```python
from build123d import *

# Parameters (mm, degrees)
SKETCH_1_W          = 22.5
SKETCH_1_H          = 17
EXTRUDE_1_DEPTH     = 6.5
SKETCH_2_W          = 7
SKETCH_2_H          = 3.2
CUT_EXTRUDE_1_DEPTH = 29.939592257
SKETCH_3_R          = 1
CUT_EXTRUDE_2_DEPTH = 2.4


with BuildPart() as part:
    # 草图1 → 凸台-拉伸1 (new body)
    with BuildSketch(Plane(origin=(0, 0, 0), x_dir=(1, 0, 0), z_dir=(0, 1, 0))):
        with Locations((11.25, 8.5)):
            Rectangle(SKETCH_1_W, SKETCH_1_H)
    extrude(amount=EXTRUDE_1_DEPTH)

    # 草图2 → 切除-拉伸1 (cut, through all)
    with BuildSketch(Plane.ZY):
        with Locations((-8.5, 1.6)):
            Rectangle(SKETCH_2_W, SKETCH_2_H)
    extrude(amount=-CUT_EXTRUDE_1_DEPTH, mode=Mode.SUBTRACT)

    # 草图3 → 切除-拉伸2 (cut)
    with BuildSketch(Plane(origin=(0, 6.5, 0), x_dir=(1, 0, 0), z_dir=(0, 1, 0))):
        with Locations(Location((7.25, 14.5, 0), (0, 0, 270))):
            Circle(SKETCH_3_R)
        with Locations(Location((15.25, 14.5, 0), (0, 0, 270))):
            Circle(SKETCH_3_R)
        with Locations(Location((15.25, 2.5, 0), (0, 0, 90))):
            Circle(SKETCH_3_R)
        with Locations(Location((7.25, 2.5, 0), (0, 0, 90))):
            Circle(SKETCH_3_R)
    extrude(amount=-CUT_EXTRUDE_2_DEPTH, mode=Mode.SUBTRACT)


solid = part.part
```
Geometry: final body of the model. Coordinates: model frame, mm. A direction names the side the tool comes from. Round coordinates to 2 decimals unless told otherwise and drop trailing zeros. Write each loop counter-clockwise with the first axis right and the second up, starting at its lowest first coordinate (ties: lowest second). Pieces come first, ordered by that corner, then holes. Notation, with made-up numbers: (74, 59) -> (94, 59) arc R28 cw to (94, 81) -> close; hole circle Ø3 at (80, 88). An arc over 180 degrees is marked (long way). Use CSV: the item, a comma, the result in double quotes. Start each with the question number.
Q1. Section D-D (x = 15.25). Return loops of the section in (y, z), plus the area to 3 significant figures.
Q2. First-contact query: pin 1 Ø2 at (x, z) = (14.5, -9) entering from -Y. Flat tip, straight axial feed; report the tip coordinate or a pass-through.
Q3. Section C-C (y = 0.75). Return loops of the section in (x, z), plus the area to 3 significant figures.
Q4. Reachability of faces 4 (the face through (15, 4.1, -2)), 5 (the face through (11, 2, -12)), 6 (the face through (11, 3, 0)) from +Z, -Z, +X, -X, +Y, -Y: full face, straight path, thin tool, end or side. Return the list, or none.
Q5. Line query: L1, parallel to X at y = 5, z = -14.5; L2, parallel to Z at x = 18.75, y = 0.75; L3, parallel to Y at x = 14.5, z = -3. Output: solid intervals per line, ascending.
Q6. Section B-B (z = -14.5). Return loops of the section in (x, y), plus the area to 3 significant figures.
Q7. Section A-A (y = 5.5). Return loops of the section in (x, z), plus the area to 3 significant figures.
Q8. Pull-direction query (X, two-part tool) for faces 1 (the face through (11, 3.2, -9)), 2 (the face through (7, 4.1, -15)), 3 (the face through (0, 4, -8)); classes: pulls with the +X half, pulls with the -X half, needs draft (parallel to the pull), parting line crosses it, or undercut.
Result sheet:
1,outline,"(0, -17) -> (6.5, -17) -> (6.5, -15.5) -> (4.1, -15.5) -> (4.1, -13.5) -> (6.5, -13.5) -> (6.5, -3.5) -> (4.1, -3.5) -> (4.1, -1.5) -> (6.5, -1.5) -> (6.5, 0) -> (0, 0) -> (0, -5) -> (3.2, -5) -> (3.2, -12) -> (0, -12) -> close"
1,area,"78.5 mm²"
2,pin 1,"y = 3.2"
3,outline,"(0, -17) -> (22.5, -17) -> (22.5, -12) -> (0, -12) -> close; (0, -5) -> (22.5, -5) -> (22.5, 0) -> (0, 0) -> close"
3,area,"225 mm²"
4,face 4,"+Y"
4,face 5,"+X, -X, -Y"
4,face 6,"+Z, +X, -X, +Y, -Y"
5,L1,"0 to 6.25, 8.25 to 14.25, 16.25 to 22.5"
5,L2,"-17 to -12, -5 to 0"
5,L3,"0 to 4.1"
6,outline,"(0, 0) -> (22.5, 0) -> (22.5, 6.5) -> (16.25, 6.5) -> (16.25, 4.1) -> (14.25, 4.1) -> (14.25, 6.5) -> (8.25, 6.5) -> (8.25, 4.1) -> (6.25, 4.1) -> (6.25, 6.5) -> (0, 6.5) -> close"
6,area,"137 mm²"
7,outline,"(0, -17) -> (22.5, -17) -> (22.5, 0) -> (0, 0) -> close; hole circle Ø2 at (7.25, -14.5); hole circle Ø2 at (7.25, -2.5); hole circle Ø2 at (15.25, -14.5); hole circle Ø2 at (15.25, -2.5)"
7,area,"370 mm²"
8,face 1,"needs draft"
8,face 2,"undercut"
8,face 3,"pulls with the -X half"
